```python
from build123d import *

# Parameters (mm, degrees)
BOSS_EXTRUDE1_DEPTH = 646.904


with BuildPart() as part:
    # Sketch1 → Boss-Extrude1 (new body)
    with BuildSketch(Plane.XY):
        Polygon((-5, -6), (-5, 6), (-9, 6), (-9, 9), (9, 9), (9, 6), (5, 6), (5, -6), (9, -6), (9, -9), (-9, -9), (-9, -6), align=None)
    extrude(amount=BOSS_EXTRUDE1_DEPTH)

    # Mirror1: part across plane


with BuildPart() as part_1:
    add(part.part)
    add(part.part.mirror(Plane(origin=(0, 0, 0), x_dir=(1, 0, 0), z_dir=(0, 0, -1))))


solid = part_1.part
```
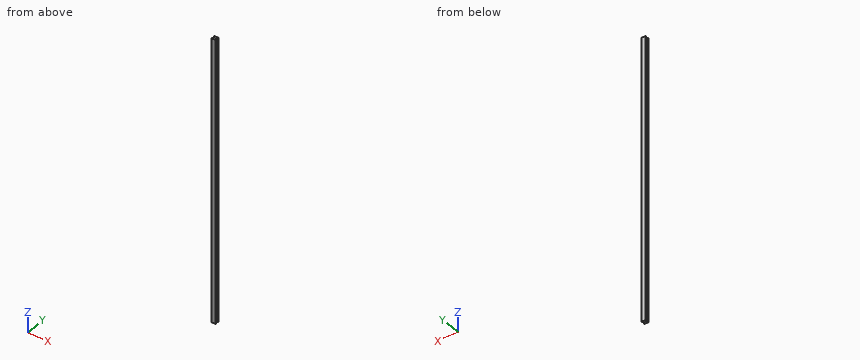
Geometry: final body of the model. Coordinates: model frame, mm. Give positions to 0.01 mm unless a question says otherwise; leave off trailing zeros. Loops run counter-clockwise (first coordinate to the right, second up) from the corner with the lowest first, then second, coordinate; pieces in that order, holes last. Notation, with made-up numbers: (76.25, -6.75) -> (96.25, -6.75) arc R19 ccw to (96.25, 17.25) -> close; hole circle Ø9 at (-24.5, 53). An arc over 180 degrees is marked (long way). Use one line per item in the form item = value.
Item 1: Section query A-A on z = -340. Output: boundary loops of the cut face in (x, y), and give its area (3 significant figures).
A:
outline = (-9, -9) -> (9, -9) -> (9, -6) -> (5, -6) -> (5, 6) -> (9, 6) -> (9, 9) -> (-9, 9) -> (-9, 6) -> (-5, 6) -> (-5, -6) -> (-9, -6) -> close
area = 228 mm^2
Item 2: Pin query (flat end, axial travel): P1, Ø6, axis at y = 2.5, z = -160, coming from the -X side; P2, Ø6, axis at y = 1.5, z = -226, coming from the +X side; P3, Ø6, axis at y = -5.5, z = -282.5, coming from the -X side. Return the tip coordinate at first contact, or that it passes through.
A:
P1 = -5
P2 = 5
P3 = -9
Item 3: Section query B-B on y = 1.5. Output: boundary loops of the cut face in (x, z).
A:
outline = (-5, -646.9) -> (5, -646.9) -> (5, 646.9) -> (-5, 646.9) -> close
Item 4: Line query: probe 1 along Y at (x, z) = (-5.5, 571); probe 2 along X at (y, z) = (3.5, -426). Output: solid intervals per line, ascending.
A:
probe_1 = -9 to -6, 6 to 9
probe_2 = -5 to 5
